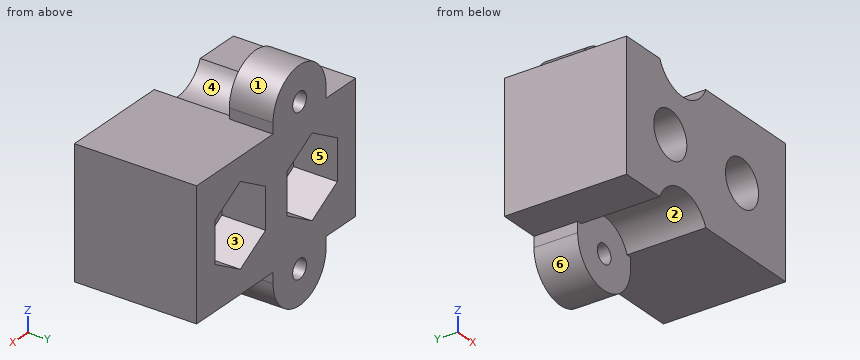
```python
from build123d import *

# Parameters (mm, degrees)
SKETCH_1_W                    = 25.5
SKETCH_1_H                    = 14.7
EXTRUDE_385_DEPTH             = 14
SKETCH_4_W                    = 8.5
SKETCH_4_H                    = 5.45
EXTRUDE_2_DEPTH               = 5
FILLET_1_RADIUS               = 4.25
FILLET_1_LENGTH               = 5
HOLE_WIZARD_M2_1_D            = 2.2
SKETCH_7_R                    = 4
CUT_EXTRUDE_3_DEPTH           = 9
FILLET_1_OF_MIRROR_1_2_RADIUS = 4.25
FILLET_1_OF_MIRROR_1_2_LENGTH = 5
HOLE_WIZARD_M5_1_D            = 5.3
CUT_EXTRUDE_4_DEPTH           = 5


with BuildPart() as part:
    # 草图1 → Extrude 385 (new body)
    with BuildSketch(Plane(origin=(0, 0, 0), x_dir=(1, 0, 0), z_dir=(0, 1, 0))):
        with Locations((16.790583128, 0)):
            Rectangle(SKETCH_1_W, SKETCH_1_H)
    extrude(amount=EXTRUDE_385_DEPTH)

    # 草图4 → 凸台-拉伸2 (add)
    with BuildSketch(Plane.XZ.offset(-14)):
        with Locations((13.040583128, -10.075)):
            Rectangle(SKETCH_4_W, SKETCH_4_H)
    extrude_2 = extrude(amount=EXTRUDE_2_DEPTH)

    # 圆角1: full round fillet: the end face becomes a half cylinder, R = half its width
    fillet_1_face = Plane((13.040583128, 11.5, -12.8), x_dir=(0, 1, 0), z_dir=(0, 0, -1))  # on the end face: x along it, z out of the body
    fillet_1_slab = fillet_1_face.offset(-FILLET_1_RADIUS / 2) * Box(FILLET_1_LENGTH, 2 * FILLET_1_RADIUS, FILLET_1_RADIUS, mode=Mode.PRIVATE)  # the body's end, R deep
    fillet_1_round = Plane((13.040583128, 11.5, -8.55), x_dir=(0, 0, -1), z_dir=(0, 1, 0)) * Cylinder(FILLET_1_RADIUS, FILLET_1_LENGTH, mode=Mode.PRIVATE)  # its axis R under the face
    add(fillet_1_slab - fillet_1_round, mode=Mode.SUBTRACT)

    # M2 间隙孔1 (through all)
    with Locations(Plane(origin=(0, 9, 0), x_dir=(-1, 0, 0), z_dir=(0, -1, 0))):
        with Locations((-13.040583128, 8.9)):
            hole_wizard_m2_1 = Hole(HOLE_WIZARD_M2_1_D / 2)

    # 草图7 → 切除-拉伸3 (cut)
    with BuildSketch(Plane.XZ):
        with Locations((13.040583128, -8.9)):
            Circle(SKETCH_7_R)
    cut_extrude_3 = extrude(amount=-CUT_EXTRUDE_3_DEPTH, mode=Mode.SUBTRACT)

    # 镜向1: 凸台-拉伸2, M2 间隙孔1, 切除-拉伸3 across plane
    add(extrude_2.mirror(Plane.XY))
    add(hole_wizard_m2_1.mirror(Plane.XY), mode=Mode.SUBTRACT)
    add(cut_extrude_3.mirror(Plane.XY), mode=Mode.SUBTRACT)

    # 圆角1 of Mirror 1 2: full round fillet: the end face becomes a half cylinder, R = half its width
    fillet_1_of_mirror_1_2_face = Plane((13.040583128, 11.5, 12.8), x_dir=(0, 1, 0), z_dir=(0, 0, 1))  # on the end face: x along it, z out of the body
    fillet_1_of_mirror_1_2_slab = fillet_1_of_mirror_1_2_face.offset(-FILLET_1_OF_MIRROR_1_2_RADIUS / 2) * Box(FILLET_1_OF_MIRROR_1_2_LENGTH, 2 * FILLET_1_OF_MIRROR_1_2_RADIUS, FILLET_1_OF_MIRROR_1_2_RADIUS, mode=Mode.PRIVATE)  # the body's end, R deep
    fillet_1_of_mirror_1_2_round = Plane((13.040583128, 11.5, 8.55), x_dir=(0, 0, 1), z_dir=(0, 1, 0)) * Cylinder(FILLET_1_OF_MIRROR_1_2_RADIUS, FILLET_1_OF_MIRROR_1_2_LENGTH, mode=Mode.PRIVATE)  # its axis R under the face
    add(fillet_1_of_mirror_1_2_slab - fillet_1_of_mirror_1_2_round, mode=Mode.SUBTRACT)

    # M5 间隙孔1 (through all)
    with Locations(Plane(origin=(0, 0, 0), x_dir=(-1, 0, 0), z_dir=(0, -1, 0))):
        with Locations((-22.540583128, 0), (-11.040583128, 0)):
            Hole(HOLE_WIZARD_M5_1_D / 2)

    # 草图10 → 切除-拉伸4 (cut)
    with BuildSketch(Plane(origin=(0, 14, 0), x_dir=(1, 0, 0), z_dir=(0, 1, 0))):
        Polygon((11.040583128, 4.67653718), (6.990583128, 2.33826859), (6.990583128, -2.33826859), (11.040583128, -4.67653718), (15.090583128, -2.33826859), (15.090583128, 2.33826859), align=None)
        Polygon((22.540583128, 4.67653718), (18.490583128, 2.33826859), (18.490583128, -2.33826859), (22.540583128, -4.67653718), (26.590583128, -2.33826859), (26.590583128, 2.33826859), align=None)
    extrude(amount=-CUT_EXTRUDE_4_DEPTH, mode=Mode.SUBTRACT)


solid = part.part
```
Geometry check sheet. Reference: the model listing, model coordinates, mm. Face numbers are marked on the shaded views. A direction names the side the tool comes from. Coordinates: 2 decimals unless noted, no trailing zeros. Order: outer loops, then holes, each group sorted by start corner. A loop starts at its lowest first (then second) coordinate and runs counter-clockwise, first axis right, second up.
Item 1: Depth check by flat-ended pin: pin 1 (1 mm diameter, centred on x = 19.5, y = 5, fed in from +Z); pin 2 (6 mm diameter, centred on x = 18.5, y = 8.5, fed in from -Z); pin 3 (1 mm diameter, centred on x = 15, z = 7.5, fed in from -Y). Enter the tip coordinate at first touch or a pass-through.
Item 2: Tool access check on the marked faces 1, 2 and 3. Record the directions out of +Z, -Z, +X, -X, +Y, -Y that give a thin tool (end or side, any length) a straight path to the whole face; none if there is none.
Item 3: Section check A-A (z = 0). Enter the section's corners in (x, y), plus the area to 3 significant figures.
Item 4: Section check C-C (y = 1.25). Enter the section's corners in (x, z), plus the area to 3 significant figures.
Item 5: Section check D-D (x = 10.5). Enter the section's corners in (y, z).
Item 6: Mould release check, pull along Z, two halves, no side actions. Record for the marked faces 4, 5 and 6: released by +Z, released by -Z, zero draft, split by the parting line, or undercut.
Item 7: Section check B-B (y = 13). Enter the section's corners in (x, z).
Item 8: Scan lines: line 1 along X through (y, z) = (7.5, 0.5); line 2 along Z through (x, y) = (5.5, 1.5); line 3 along Y through (x, z) = (13, -11). Record each from-to range of solid material in increasing order.
Check sheet entries:
1. pin 1: stops at z = 7.35
1. pin 2: stops at z = -11.99
1. pin 3: stops at y = 9
2. face 1: +Z, +Y, -Y
2. face 2: -Z, -Y
2. face 3: +Y
3. outline: (4.04, 0) - (8.39, 0) - (8.39, 9) - (6.99, 9) - (6.99, 14) - (4.04, 14) - close; (13.69, 0) - (19.89, 0) - (19.89, 9) - (18.49, 9) - (18.49, 14) - (15.09, 14) - (15.09, 9) - (13.69, 9) - close; (25.19, 0) - (29.54, 0) - (29.54, 14) - (26.59, 14) - (26.59, 9) - (25.19, 9) - close
3. area: 181 mm2
4. outline: (4.04, -7.35) - (9.35, -7.35) arc R4 cw to (16.73, -7.35) - (29.54, -7.35) - (29.54, 7.35) - (16.73, 7.35) arc R4 cw to (9.35, 7.35) - (4.04, 7.35) - close; hole circle Ø5.3 at (11.04, 0); hole circle Ø5.3 at (22.54, 0)
4. area: 305 mm2
5. outline: (0, -5.81) - (9, -5.81) - (9, -11.96) - (14, -11.96) - (14, -4.36) - (9, -4.36) - (9, -2.59) - (0, -2.59) - close; (0, 2.59) - (9, 2.59) - (9, 4.36) - (14, 4.36) - (14, 11.96) - (9, 11.96) - (9, 5.81) - (0, 5.81) - close
6. face 4: released by +Z
6. face 5: undercut
6. face 6: released by -Z
7. outline: (4.04, -7.35) - (8.79, -7.35) - (8.79, -8.55) arc R4.25 ccw to (17.29, -8.55) - (17.29, -7.35) - (29.54, -7.35) - (29.54, 7.35) - (17.29, 7.35) - (17.29, 8.55) arc R4.25 ccw to (8.79, 8.55) - (8.79, 7.35) - (4.04, 7.35) - close; hole (6.99, -2.34) - (11.04, -4.68) - (15.09, -2.34) - (15.09, 2.34) - (11.04, 4.68) - (6.99, 2.34) - close; hole circle Ø2.2 at (13.04, -8.9); hole circle Ø2.2 at (13.04, 8.9); hole (18.49, -2.34) - (22.54, -4.68) - (26.59, -2.34) - (26.59, 2.34) - (22.54, 4.68) - (18.49, 2.34) - close
8. line 1: x = 4.04 to 8.44, 13.64 to 19.94, 25.14 to 29.54
8. line 2: z = -7.35 to 7.35
8. line 3: y = 9 to 14
